For this review, take the finished solid that the model builds, in its own axes (mm). A direction names the side the tool comes from. Coordinates: 2 decimals unless noted, no trailing zeros. Order: outer loops, then holes, each group sorted by start corner. A loop starts at its lowest first (then second) coordinate and runs counter-clockwise, first axis right, second up. Notation, with made-up numbers: (-5.75, -22) -> (17.25, -22) arc R35 cw to (17.25, 14) -> close; hole circle Ø1 at (12.25, 12). An arc over 180 degrees is marked (long way). Answer as a JSON object with one key per item and string values. Group by question number.
1) Wall thickness on L1, parallel to X at y = -384, z = 2; L2, parallel to Y at x = 39.5, z = 7; L3, parallel to Y at x = -216, z = 14.25: over which ranges is each line inside the solid? List them lowest first.
2) Machinability: for faces 1 (the flat face through (-541.723, -158, 9)), 2 (the flat face through (-509.973, -197, 9)), which of the approach directions +Z, -Z, +X, -X, +Y, -Y give a long, thin tool a straight path to every point of the face, cutting with its end or side? Answer none if there is none.
3) Add section B-B, the plane x = -502. Write out the cut boundary in (y, z), then the cut area to 3 significant figures.
4) Add section C-C, the plane z = 8.25. Write out the cut boundary in (x, y).
5) Draft analysis for pull direction Y (two halves, no side actions). For faces 3 (the flat face through (-232.66, -451.28, 9.39)), 4 (the flat face through (-491.045, -362, 9)), 5 (the flat face through (67.877, -158, 9)), 6 (the flat face through (42.599, -362, 9)), state which applies: +Y half, -Y half, draft (parallel to the pull), parting line (faces both ways), or undercut.
6) For pin 1 (6 mm diameter, centred on x = -432, y = 85.5, fed in from -Z); pin 2 (5.5 mm diameter, centred on x = 33, z = 9.5, fed in from -Y); pin 3 (2 mm diameter, centred on x = -277.5, z = 8.5, fed in from -Y); pin 4 (2 mm diameter, centred on x = -285, z = 5, fed in from -Y), all flat-tipped, find the tip position at first contact; note any pin that passes through.
7) Add section A-A, the plane y = -174. Write out the cut boundary in (x, z), then the cut area to 3 significant figures.
from build123d import *

# Parameters (mm, degrees)
F0_W     = 609.6
F0_H     = 609.6
F1_DEPTH = 19.05
F4_DEPTH = 747.014
F2_W     = 19.05
F2_H     = 76.2
F5_DEPTH = 25.4


with BuildPart() as f1:
    # F0 (on Top) → F1 (new body)
    with BuildSketch(Plane.XY):
        with Locations((-236.922948, -153.95108)):
            Rectangle(F0_W, F0_H)
    extrude(amount=F1_DEPTH)

    # F3 (on face) → F4 (cut)
    with BuildSketch(Plane.YZ.offset(67.877052)):
        Polygon((-444.019914, 0), (-458.75108, 19.05), (-458.75108, 0), align=None)
    extrude(amount=-F4_DEPTH, mode=Mode.SUBTRACT)

    # F2 (on face) → F5 (cut)
    with BuildSketch(Plane(origin=(0, 0, 0), x_dir=(1, 0, 0), z_dir=(0, 0, -1))):
        with Locations((-500.570309, 362.360354)):
            Rectangle(F2_W, F2_H)
        with Locations((-500.447948, 197.260354)):
            Rectangle(F2_W, F2_H)
        with Locations((32.952052, 197.260354)):
            Rectangle(F2_W, F2_H)
        with Locations((33.074412, 362.360354)):
            Rectangle(F2_W, F2_H)
    extrude(amount=-F5_DEPTH, mode=Mode.SUBTRACT)


solid = f1.part
Output values:
{
 "1": {"L1": "x = -541.72 to -510.1, -491.05 to 23.55, 42.6 to 67.88", "L2": "y = -449.43 to -400.46, -324.26 to -235.36, -159.16 to 150.85", "L3": "y = -455.04 to 150.85"},
 "2": {"face 1": "+Z, -Z, -X, +Y, -Y", "face 2": "+Z, -Z"},
 "3": {"outline": "(-458.75, 19.05) -> (-444.02, 0) -> (-400.46, 0) -> (-400.46, 19.05) -> close; (-324.26, 0) -> (-235.36, 0) -> (-235.36, 19.05) -> (-324.26, 19.05) -> close; (-159.16, 0) -> (150.85, 0) -> (150.85, 19.05) -> (-159.16, 19.05) -> close", "area": "8,570 mm²"},
 "4": {"outline": "(-541.72, -450.4) -> (67.88, -450.4) -> (67.88, 150.85) -> (-541.72, 150.85) -> close; hole (-510.1, -400.46) -> (-491.05, -400.46) -> (-491.05, -324.26) -> (-510.1, -324.26) -> close; hole (-509.97, -235.36) -> (-490.92, -235.36) -> (-490.92, -159.16) -> (-509.97, -159.16) -> close; hole (23.43, -235.36) -> (42.48, -235.36) -> (42.48, -159.16) -> (23.43, -159.16) -> close; hole (23.55, -400.46) -> (42.6, -400.46) -> (42.6, -324.26) -> (23.55, -324.26) -> close"},
 "5": {"face 3": "-Y half", "face 4": "undercut", "face 5": "draft", "face 6": "undercut"},
 "6": {"pin 1": "stops at z = 0", "pin 2": "stops at y = -453.49", "pin 3": "stops at y = -451.37", "pin 4": "stops at y = -448.66"},
 "7": {"outline": "(-541.72, 0) -> (-509.97, 0) -> (-509.97, 19.05) -> (-541.72, 19.05) -> close; (-490.92, 0) -> (23.43, 0) -> (23.43, 19.05) -> (-490.92, 19.05) -> close; (42.48, 0) -> (67.88, 0) -> (67.88, 19.05) -> (42.48, 19.05) -> close", "area": "10,900 mm²"}
}
